Check sheet for the drawn part. Datum: minimum x, y, z corner. Units: mm. A direction names the side the tool comes from. Round coordinates to 2 decimals unless told otherwise and drop trailing zeros. Write each loop counter-clockwise with the first axis right and the second up, starting at its lowest first coordinate (ties: lowest second). Pieces come first, ordered by that corner, then holes. Notation, with made-up numbers: (-23, -27) -> (19, -27) arc R27 cw to (19, -11) -> close; hole circle Ø5 at (37.5, 48.25). An arc over 180 degrees is marked (long way). One line per item, written item: value.
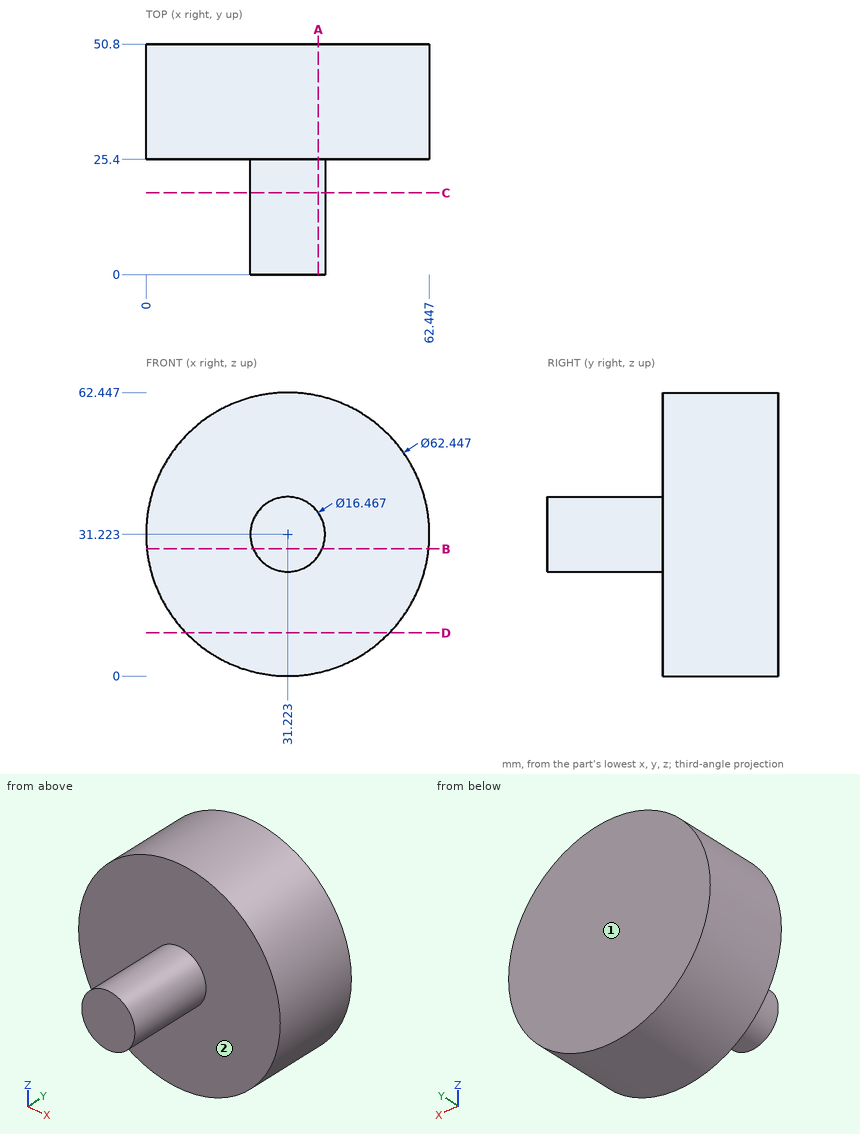
Item 1: Sectioned sample at A-A on x = 38. Enter the section's corners in (y, z) (1 decimal).
Answer:
outline: (0, 26.5) -> (25.4, 26.5) -> (25.4, 0.7) -> (50.8, 0.7) -> (50.8, 61.7) -> (25.4, 61.7) -> (25.4, 35.9) -> (0, 35.9) -> close
Item 2: Sectioned sample at C-C on y = 18. Enter the section's corners in (x, z), and give its area (3 significant figures).
Answer:
outline: circle Ø16.47 at (31.22, 31.22)
area: 213 mm^2
Item 3: Depth check by flat-ended pin: P1, Ø12, axis at x = 17, y = 37.5, coming from the -Z side; P2, Ø10, axis at x = 50, y = 39, coming from the -Z side. Enter the tip coordinate at first touch or a pass-through.
Answer:
P1: stops at z = 1.1
P2: stops at z = 3.2
Item 4: Tool access check on the marked faces 1 and 2. Record the directions out of +Z, -Z, +X, -X, +Y, -Y that give a thin tool (end or side, any length) a straight path to the whole face; none if there is none.
Answer:
face 1: +Z, -Z, +X, -X, +Y
face 2: -Y
Item 5: Thickness scan on line 1 (Y direction, x = 36, z = 60.5); line 2 (Z direction, x = 19.5, y = 30) (1 decimal); line 3 (Z direction, x = 31, y = 45). Record the ranges inside material, lowest first.
Answer:
line 1: y = 25.4 to 50.8
line 2: z = 2.3 to 60.2
line 3: z = 0 to 62.45
Item 6: Sectioned sample at D-D on z = 9.5. Enter the section's corners in (x, y), and give its area (3 significant figures).
Answer:
outline: (8.8, 25.4) -> (53.65, 25.4) -> (53.65, 50.8) -> (8.8, 50.8) -> close
area: 1,140 mm^2
Item 7: Sectioned sample at B-B on z = 28. Enter the section's corners in (x, y).
Answer:
outline: (0.17, 25.4) -> (23.65, 25.4) -> (23.65, 0) -> (38.8, 0) -> (38.8, 25.4) -> (62.28, 25.4) -> (62.28, 50.8) -> (0.17, 50.8) -> close
